Geometry: final body of the model. Coordinates: model frame, mm. Give positions to 0.01 mm unless a question says otherwise; leave off trailing zeros. Write each loop counter-clockwise with the first axis right and the second up, starting at its lowest first coordinate (ties: lowest second). Pieces come first, ordered by that corner, then holes.
```python
from build123d import *


with BuildPart() as f2:
    # F0 (on Top) → F2 (revolve)
    with BuildSketch(Plane.XY):
        with BuildLine():
            Line((0, -42.264973081), (0, 157.735026919))
            ThreePointArc((0, 157.735026919), (-100, 57.735026919), (0, -42.264973081))
        make_face()
    revolve(axis=Axis((0, 57.735026919, 0), (0, -1, 0)))


with BuildPart() as f3_1:
    # F3: copy of F2
    add(f2.part.moved(Location((-50, -86.6025403784, 0))))


with BuildPart() as f4_1:
    # F4: copy of F2
    add(f2.part.moved(Location((50, -86.6025403784, 0))))


with BuildPart() as f5_1:
    # F5: copy of F2
    add(f2.part.moved(Location((0, -57.735026919, 81.6496580928))))


with BuildPart() as f2_1:
    add(f2.part)

    # F6: intersect F3_1, F4_1, F5_1
    add(f3_1.part, mode=Mode.INTERSECT)
    add(f4_1.part, mode=Mode.INTERSECT)
    add(f5_1.part, mode=Mode.INTERSECT)


solid = f2_1.part
```
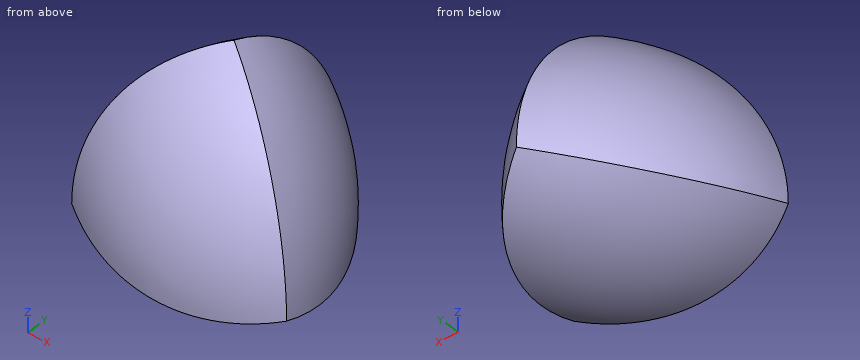
Item 1: Section C-C, the plane z = -7. Return the cut outline in (x, y).
Found:
outline: (-46.21, -2.5) arc R46.27 ccw to (-25.27, -38.77) arc R99.75 ccw to (25.27, -38.77) arc R46.27 ccw to (46.21, -2.5) arc R99.75 ccw to (20.94, 41.26) arc R46.27 ccw to (-20.94, 41.26) arc R99.75 ccw to start
Item 2: Section A-A, the plane x = -16.5. Return the cut outline in (y, z), plus the area to 3 significant figures.
Found:
outline: (-40.55, -8.26) arc R98.63 ccw to (45.59, -5.81) arc R74.68 ccw to (-9.53, 72.14) arc R98.63 ccw to start
area: 5,700 mm2
Item 3: Pin query (flat end, axial travel): pin 1 Ø5 at (x, y) = (-22.5, -1.5) entering from -Z; pin 2 Ø3 at (x, z) = (-5, 22) entering from -Y; pin 3 Ø1 at (x, y) = (16.5, 25) entering from +Z. Return the tip coordinate at first contact, or that it passes through.
Found:
pin 1: stops at z = -16.32
pin 2: stops at y = -40.02
pin 3: stops at z = 52.55
Item 4: Line query: L1, parallel to Z at x = 36.5, y = -11; L2, parallel to Z at x = 37, y = -14; L3, parallel to Y at x = -25.5, z = 27.5. Output: solid intervals per line, ascending.
Found:
L1: z = -10.8 to 46.89
L2: z = -10.19 to 47.01
L3: y = -34.97 to 30.66
Item 5: Section D-D, the plane x = 16. Return the cut outline in (y, z).
Found:
outline: (-40.63, -8.31) arc R98.71 ccw to (46.05, -5.66) arc R75.13 ccw to (-9.24, 72.52) arc R98.71 ccw to start
